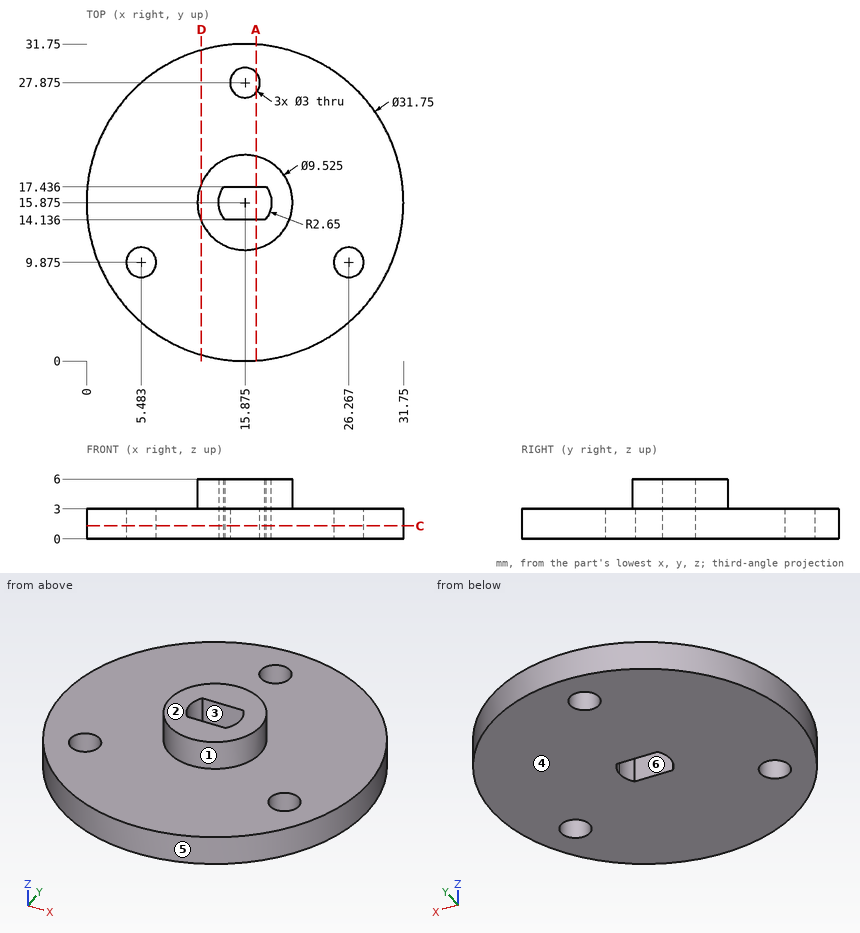
Part print with two shaded views. Sizes in mm from the minimum x, y, z corner. A direction names the side the tool comes from. Round coordinates to 2 decimals unless told otherwise and drop trailing zeros. Write each loop counter-clockwise with the first axis right and the second up, starting at its lowest first coordinate (ties: lowest second). Pieces come first, ordered by that corner, then holes. Notation, with made-up numbers: M 65,64 L 96,64 A11 cw 96,76 Z; hole C 72,35 d3. An arc over 180 degrees is marked long. Answer as CSV lines item,"result". Start each with the question number.
1) Which spindle directions (+Z, -Z, +X, -X, +Y, -Y) get a long thin tool onto all of the face, cutting with end or side? Do the marked faces 1, 2 and 3. Say none if no direction does.
2) Drop flat-ended pins along their axis: pin 1 (3.5 mm diameter, centred on x = 15.875, y = 27.875, fed in from -Z); pin 2 (5 mm diameter, centred on x = 5.48, y = 9.88, fed in from +Z); pin 3 (1 mm diameter, centred on y = 17.5, z = 5, fed in from +X); pin 4 (1 mm diameter, centred on y = 26, z = 3, fed in from +X). Give the stop position or say it passes through.
3) Drill centre lines: L1, parallel to Y at x = 17, z = 0.3 (1 decimal); L2, parallel to Z at x = 3, y = 20; L3, parallel to Y at x = 15.5, z = 1.15 (1 decimal). Where is each one in solid material? Low to high.
4) Mould opens along X. For the marked faces 4, 5 and 6 say: +X half, -X half, draft (parallel to the pull), parting line (faces both ways), or undercut.
5) Band-saw the part on C-C (z = 1.3). Count the separate pieces of the cut face and the enclosed holes in it, then the cut area to 3 significant figures.
6) Band-saw the part on A-A (x = 17). List the corners of the cut face in (y, z).
7) Band-saw the part on D-D (x = 11.5). List the corners of the cut face in (y, z) (1 decimal).
Worked out:
1,face 1,"+Z"
1,face 2,"+Z, +X, -X, +Y, -Y"
1,face 3,"+Z, -Z"
2,pin 1,"z = 0"
2,pin 2,"z = 3"
2,pin 3,"x = 20.5"
2,pin 4,"x = 28.5"
3,L1,"0 to 14.1, 17.4 to 26.9, 28.9 to 31.7"
3,L2,"0 to 3"
3,L3,"0 to 14.1, 17.4 to 26.4, 29.3 to 31.7"
4,face 4,"draft"
4,face 5,"parting line"
4,face 6,"undercut"
5,separate pieces,"1"
5,enclosed holes,"4"
5,area,"754 mm²"
6,outline,"M 0.04,0 L 14.14,0 L 14.14,6 L 11.25,6 L 11.25,3 L 0.04,3 Z; M 17.44,0 L 26.88,0 L 26.88,3 L 20.5,3 L 20.5,6 L 17.44,6 Z; M 28.87,0 L 31.71,0 L 31.71,3 L 28.87,3 Z"
7,outline,"M 0.6,0 L 31.1,0 L 31.1,3 L 17.8,3 L 17.8,6 L 14,6 L 14,3 L 0.6,3 Z"
